```python
from build123d import *

# Parameters (mm, degrees)
ESQUISSE1_W        = 2
ESQUISSE1_H        = 2
BOSS_EXTRU_1_DEPTH = 2
CONG_1_R           = 1.2


with BuildPart() as part:
    # Esquisse1 → Boss.-Extru.1 (new body)
    with BuildSketch(Plane.XY):
        with BuildLine():
            Line((2.198395722, -3.372264328), (0.598395722, -3.372264328))
            Line((0.598395722, -3.372264328), (0.598395722, -16.322874175))
            ThreePointArc((0.598395722, -16.322874175), (1.398395722, -16.172264328), (2.198395722, -16.322874175))
            Line((2.198395722, -16.322874175), (2.198395722, -3.372264328))
        make_face()
        Polygon((-0.601604278, -1.372264328), (-1.601604278, -1.372264328), (0.598395722, -3.372264328), (2.198395722, -3.372264328), (4.398395722, -1.372264328), (3.398395722, -1.372264328), (1.398395722, -1.372264328), align=None)
        with Locations((2.398395722, -0.372264328)):
            Rectangle(ESQUISSE1_W, ESQUISSE1_H)
        with Locations((0.398395722, -0.372264328)):
            Rectangle(ESQUISSE1_W, ESQUISSE1_H)
        with BuildLine():
            ThreePointArc((2.198395722, -16.322874175), (1.398395722, -16.172264328), (0.598395722, -16.322874175))
            Line((0.598395722, -16.322874175), (0.598395722, -17.411795692))
            ThreePointArc((0.598395722, -17.411795692), (1.398395722, -17.122264328), (2.198395722, -17.411795692))
            Line((2.198395722, -17.411795692), (2.198395722, -16.322874175))
        make_face()
        with BuildLine():
            Line((0.598395722, -17.411795692), (0.598395722, -16.322874175))
            ThreePointArc((0.598395722, -16.322874175), (0.157428357, -20.188854541), (3.598395722, -18.372264328))
            ThreePointArc((3.598395722, -18.372264328), (3.214985934, -17.131296963), (2.198395722, -16.322874175))
            Line((2.198395722, -16.322874175), (2.198395722, -17.411795692))
            ThreePointArc((2.198395722, -17.411795692), (2.530318864, -17.841934242), (2.648395722, -18.372264328))
            ThreePointArc((2.648395722, -18.372264328), (0.868065636, -19.50418747), (0.598395722, -17.411795692))
        make_face()
    extrude(amount=BOSS_EXTRU_1_DEPTH)

    # Congé1
    cong_1_edges = [part.edges().sort_by_distance(p)[0] for p in [
        (2.198395722, -16.322874175, 1),
        (0.598395722, -16.322874175, 1),
    ]]
    fillet(cong_1_edges, radius=CONG_1_R)


solid = part.part
```
CAD build for the part. Positions are in the model's coordinates, mm. A direction names the side the tool comes from. Round coordinates to 2 decimals unless told otherwise and drop trailing zeros. Order: outer loops, then holes, each group sorted by start corner. A loop starts at its lowest first (then second) coordinate and runs counter-clockwise, first axis right, second up.
Item 1: Saw through at C-C on y = -19. Write the cut outline in (x, z).
Item 2: Pin check, flat tips, straight feed: pin 1 (0.5 mm diameter, centred on x = 4, z = 1, fed in from +Y); pin 2 (0.6 mm diameter, centred on y = -1, z = 1, fed in from +X); pin 3 (1.5 mm diameter, centred on x = -1, y = -15.5, fed in from +Z). Stop position of each tip, or through.
Item 3: Probe line 1 along Y through (x, z) = (1.35, 0.8); line 2 along X through (y, z) = (-10.25, 1.85); line 3 along Y through (x, z) = (0.9, 1.5). List the from-to ranges inside material, lowest first.
Item 4: Tool access for faces 4 (the face through (-1, -1.372, 1)), 5 (the face through (0.598, -9, 1)), 6 (the face through (3.28, -2.39, 0.99)), 7 (the face through (3.398, 0, 1)), 8 (the face through (1, -10, 0)): list every direction of +Z, -Z, +X, -X, +Y, -Y with a clear straight run to the whole face (end or side of a thin tool).
Item 5: Saw through at B-B on z = 1.3. Write the cut outline in (x, y).
Item 6: Saw through at D-D on y = -6. Write the cut outline in (x, z).
Item 7: Saw through at A-A on x = 1.2. Write the cut outline in (y, z).
Item 8: Mould opens along Y. For faces 1 (the face through (-0.602, 0, 1)), 2 (the face through (1, 0.628, 1)), 3 (the face through (2.33, -16.17, 1.01)) say: pulls with the +Y half, pulls with the -Y half, needs draft (parallel to the pull), parting line crosses it, or undercut.
Reported:
1. outline: (-0.71, 0) - (0.32, 0) - (0.32, 2) - (-0.71, 2) - close; (2.48, 0) - (3.51, 0) - (3.51, 2) - (2.48, 2) - close
2. pin 1: stops at y = -1.37
2. pin 2: stops at x = 3.4
2. pin 3: passes through
3. line 1: y = -20.57 to -19.62, -17.12 to 0.63
3. line 2: x = 0.6 to 2.2
3. line 3: y = -20.52 to -19.52, -17.23 to 0.63
4. face 4: +Z, -Z, -X, +Y
4. face 5: +Z, -Z, -X
4. face 6: +Z, -Z, +X
4. face 7: +Z, -Z, +X, +Y
4. face 8: -Z, +X, -X, +Y, -Y
5. outline: (-1.6, -1.37) - (0.6, -3.37) - (0.6, -15.62) arc R1.2 cw to (0.1, -16.59) arc R2.2 ccw (long way) to (2.69, -16.59) arc R1.2 cw to (2.2, -15.62) - (2.2, -3.37) - (4.4, -1.37) - (3.4, -1.37) - (3.4, 0.63) - (-0.6, 0.63) - (-0.6, -1.37) - close; hole circle Ø2.5 at (1.4, -18.37)
6. outline: (0.6, 0) - (2.2, 0) - (2.2, 2) - (0.6, 2) - close
7. outline: (-20.56, 0) - (-19.61, 0) - (-19.61, 2) - (-20.56, 2) - close; (-17.14, 0) - (0.63, 0) - (0.63, 2) - (-17.14, 2) - close
8. face 1: needs draft
8. face 2: pulls with the +Y half
8. face 3: undercut
